from build123d import *

# Parameters (mm, degrees)
SKETCH_1_W          = 95.5
SKETCH_1_H          = 95.5
EXTRUDE_1_DEPTH     = 12
CUT_EXTRUDE_1_DEPTH = 69.58662406
FILLET_2_R          = 15
SKETCH_3_R          = 75
EXTRUDE_2_DEPTH     = 2
CHAMFER_1_SIZE      = 12
FILLET_1_R          = 1
SKETCH_6_W          = 42
SKETCH_6_H          = 42
CUT_EXTRUDE_3_DEPTH = 107.98598046
SKETCH_7_R          = 1.6
CUT_EXTRUDE_4_DEPTH = 107.98598046
CUT_EXTRUDE_5_DEPTH = 107.98598046
CUT_EXTRUDE_6_DEPTH = 0.5
SKETCH_10_W         = 12
SKETCH_10_H         = 12
CUT_EXTRUDE_7_DEPTH = 107.98598046
SKETCH_11_W         = 42
SKETCH_11_H         = 42
EXTRUDE_3_DEPTH     = 14
FILLET_3_R          = 2
SKETCH_12_W         = 41.3
SKETCH_12_H         = 41.3
CUT_EXTRUDE_8_DEPTH = 107.98598046
FILLET_4_R          = 5
SKETCH_13_R         = 3.25
CUT_EXTRUDE_9_DEPTH = 3


with BuildPart() as part:
    # ｽｹｯﾁ1 → ﾎﾞｽ - 押し出し1 (new body)
    with BuildSketch(Plane.XY):
        Rectangle(SKETCH_1_W, SKETCH_1_H)
    extrude(amount=EXTRUDE_1_DEPTH)

    # ｽｹｯﾁ2 → ｶｯﾄ - 押し出し1 (cut, through all)
    with BuildSketch(Plane.XY.offset(12)):
        Polygon((-16, 47.75), (-20, 20), (-47.75, 16), (-47.75, 47.75), align=None)
        Polygon((-16, -47.75), (-20, -20), (-47.75, -16), (-47.75, -47.75), align=None)
    cut_extrude_1 = extrude(amount=-CUT_EXTRUDE_1_DEPTH, mode=Mode.SUBTRACT)

    # ﾐﾗｰ1: ｶｯﾄ - 押し出し1 across plane
    add(cut_extrude_1.mirror(Plane(origin=(0, 0, 0), x_dir=(0, 0, 1), z_dir=(1, 0, 0))), mode=Mode.SUBTRACT)

    # ﾌｨﾚｯﾄ2
    fillet_2_edges = [part.edges().sort_by_distance(p)[0] for p in [
        (-20, 20, 6),
        (-20, -20, 6),
        (20, 20, 6),
        (20, -20, 6),
    ]]
    fillet(fillet_2_edges, radius=FILLET_2_R)

    # ｽｹｯﾁ3 → ﾎﾞｽ - 押し出し2 (add)
    with BuildSketch(Plane(origin=(0, 0, 0), x_dir=(-1, 0, 0), z_dir=(0, 0, -1))):
        Circle(SKETCH_3_R)
    extrude(amount=EXTRUDE_2_DEPTH)

    # 面取り1
    chamfer_1_edges = [part.edges().sort_by_distance(p)[0] for p in [
        (0, 47.75, 0),
        (47.75, 0, 0),
        (0, -47.75, 0),
        (-47.75, 0, 0),
    ]]
    chamfer(chamfer_1_edges, length=CHAMFER_1_SIZE - 0.0001)  # a hair under: the kernel refuses the full size

    # ﾌｨﾚｯﾄ1
    fillet_1_edges = [part.edges().sort_by_distance(p)[0] for p in [
        (75, 0, 0),
        (75, 0, -2),
    ]]
    fillet(fillet_1_edges, radius=FILLET_1_R - 0.0001)  # a hair under: the kernel refuses the full size

    # ｽｹｯﾁ6 → ｶｯﾄ - 押し出し3 (cut, through all)
    with BuildSketch(Plane.XY.offset(12)):
        Rectangle(SKETCH_6_W, SKETCH_6_H)
    extrude(amount=-CUT_EXTRUDE_3_DEPTH, mode=Mode.SUBTRACT)

    # ｽｹｯﾁ7 → ｶｯﾄ - 押し出し4 (cut, through all)
    with BuildSketch(Plane.XY.offset(12)):
        with Locations((0.15, 39.15)):
            Circle(SKETCH_7_R)
        with Locations((-39.15, 0.15)):
            Circle(SKETCH_7_R)
        with Locations((39.15, -0.15)):
            Circle(SKETCH_7_R)
        with Locations((-0.15, -39.15)):
            Circle(SKETCH_7_R)
    extrude(amount=-CUT_EXTRUDE_4_DEPTH, mode=Mode.SUBTRACT)

    # ｽｹｯﾁ8 → ｶｯﾄ - 押し出し5 (cut, through all)
    with BuildSketch(Plane(origin=(0, 0, -2), x_dir=(-1, 0, 0), z_dir=(0, 0, -1))):
        Polygon((-45.748737342, 53.526911935), (-46.809397513, 52.466251763), (-45.04163056, 50.69848481), (-43.980970389, 51.759144982), align=None)
        Polygon((-53.526911935, 45.748737342), (-51.759144982, 43.980970389), (-50.69848481, 45.04163056), (-52.466251763, 46.809397513), align=None)
        Polygon((43.980970389, 51.759144982), (45.04163056, 50.69848481), (46.809397513, 52.466251763), (45.748737342, 53.526911935), align=None)
        Polygon((51.759144982, 43.980970389), (53.526911935, 45.748737342), (52.466251763, 46.809397513), (50.69848481, 45.04163056), align=None)
    cut_extrude_5 = extrude(amount=-CUT_EXTRUDE_5_DEPTH, mode=Mode.SUBTRACT)

    # ｽｹｯﾁ9 → ｶｯﾄ - 押し出し6 (cut)
    with BuildSketch(Plane.XY):
        Polygon((-53.526911935, 45.748737342), (-45.748737342, 53.526911935), (-43.980970389, 51.759144982), (-51.759144982, 43.980970389), align=None)
        Polygon((43.980970389, 51.759144982), (51.759144982, 43.980970389), (53.526911935, 45.748737342), (45.748737342, 53.526911935), align=None)
    cut_extrude_6 = extrude(amount=-CUT_EXTRUDE_6_DEPTH, mode=Mode.SUBTRACT)

    # ﾐﾗｰ2: ｶｯﾄ - 押し出し5, ｶｯﾄ - 押し出し6 across plane
    add(cut_extrude_5.mirror(Plane.ZX), mode=Mode.SUBTRACT)
    add(cut_extrude_6.mirror(Plane.ZX), mode=Mode.SUBTRACT)

    # ｽｹｯﾁ10 → ｶｯﾄ - 押し出し7 (cut, through all)
    with BuildSketch(Plane.XY.offset(12)):
        with Locations((-29.75, 9.25)):
            Rectangle(SKETCH_10_W, SKETCH_10_H)
        with Locations((-9.25, -29.75)):
            Rectangle(SKETCH_10_W, SKETCH_10_H)
        with Locations((29.75, -9.25)):
            Rectangle(SKETCH_10_W, SKETCH_10_H)
        with Locations((9.25, 29.75)):
            Rectangle(SKETCH_10_W, SKETCH_10_H)
    extrude(amount=-CUT_EXTRUDE_7_DEPTH, mode=Mode.SUBTRACT)

    # ｽｹｯﾁ11 → ﾎﾞｽ - 押し出し3 (add, through all)
    with BuildSketch(Plane(origin=(0, 0, -2), x_dir=(-1, 0, 0), z_dir=(0, 0, -1))):
        Rectangle(SKETCH_11_W, SKETCH_11_H)
    extrude(amount=-EXTRUDE_3_DEPTH)

    # ﾌｨﾚｯﾄ3
    fillet_3_edges = [part.edges().sort_by_distance(p)[0] for p in [
        (-35.75, 3.25, 5),
        (-35.75, 15.25, 5),
        (-23.75, 15.25, 5),
        (-23.75, 3.25, 5),
        (-15.25, -35.75, 5),
        (-15.25, -23.75, 5),
        (-3.25, -23.75, 5),
        (-3.25, -35.75, 5),
        (35.75, -3.25, 5),
        (35.75, -15.25, 5),
        (23.75, -15.25, 5),
        (23.75, -3.25, 5),
        (15.25, 35.75, 5),
        (15.25, 23.75, 5),
        (3.25, 23.75, 5),
        (3.25, 35.75, 5),
    ]]
    fillet(fillet_3_edges, radius=FILLET_3_R)

    # ｽｹｯﾁ12 → ｶｯﾄ - 押し出し8 (cut, through all)
    with BuildSketch(Plane.XY.offset(12)):
        Rectangle(SKETCH_12_W, SKETCH_12_H)
    extrude(amount=-CUT_EXTRUDE_8_DEPTH, mode=Mode.SUBTRACT)

    # ﾌｨﾚｯﾄ4
    fillet_4_edges = [part.edges().sort_by_distance(p)[0] for p in [
        (-20.65, -20.65, 5),
        (-20.65, 20.65, 5),
        (20.65, 20.65, 5),
        (20.65, -20.65, 5),
    ]]
    fillet(fillet_4_edges, radius=FILLET_4_R)

    # ｽｹｯﾁ13 → ｶｯﾄ - 押し出し9 (cut)
    with BuildSketch(Plane(origin=(0, 0, -2), x_dir=(-1, 0, 0), z_dir=(0, 0, -1))):
        with Locations((-0.15, 39.15)):
            Circle(SKETCH_13_R)
        with Locations((39.15, 0.15)):
            Circle(SKETCH_13_R)
        with Locations((-39.15, -0.15)):
            Circle(SKETCH_13_R)
        with Locations((0.15, -39.15)):
            Circle(SKETCH_13_R)
    extrude(amount=-CUT_EXTRUDE_9_DEPTH, mode=Mode.SUBTRACT)


solid = part.part
The listing builds one solid part. Answer for the finished solid, in the listing's coordinates (mm). A direction names the side the tool comes from. Coordinates: 2 decimals unless noted, no trailing zeros. Answer in a Markdown table with one row per item. Add a question column.
1. Determine the mould class of faces 4 (the flat face through (-22, 1, 12)), 5 (the flat face through (-9, -35.75, 5)), 6 (the flat face through (53.67, -0.22, 6.08)) for opening direction X: +X half, -X half, draft (parallel to the pull), parting line (faces both ways), or undercut.
2. The part is cut by section A-A, the plane y = -11. Count the separate pieces of the cut face and the enclosed holes in it, then the cut area to 3 significant figures.
3. For faces 1 (the cylindrical face through (-3.25, -38.17, -0.52)), 2 (the cylindrical face through (-22.735, -22.544, 5.916)), 3 (the flat face through (9, 23.75, 5)), determine the directions among +Z, -Z, +X, -X, +Y, -Y from which every point of the face is accessible in a straight line to the end or side of a thin tool.
4. Flat-ended cylindrical pins translate along their axes: P1, Ø6.5, axis at x = 28, z = 5.5, coming from the -Y side; P2, Ø8, axis at y = 53.5, z = 7.5, coming from the -X side; P3, Ø7, axis at x = -38, y = 0.5, coming from the -Z side; P4, Ø6.5, axis at y = -10.5, z = 7.5, coming from the +X side. Find the tip coordinate at first contact, or state that the pin passes through.
5. Consider line 1 (Y direction, x = 0.15, z = 5); line 2 (Y direction, x = 53, z = -0.25); line 3 (Y direction, x = 0.15, z = 6.5). Determine where each line is inside the solid, lowest interval first. Write a range as [from, to].
Answer below:
| question | item | result |
|---|---|---|
| 1 | face 4 | draft |
| 1 | face 5 | undercut |
| 1 | face 6 | +X half |
| 2 | separate pieces | 3 |
| 2 | enclosed holes | 0 |
| 2 | area | 840 mm2 |
| 3 | face 1 | -Z |
| 3 | face 2 | +Z, -X, -Y |
| 3 | face 3 | +Z, -Z |
| 4 | P1 | y = -20.88 |
| 4 | P2 | x = -15.75 |
| 4 | P3 | z = -2 |
| 4 | P4 | x = 55.5 |
| 5 | line 1 | [-54.75, -40.72], [-37.58, -20.65], [20.65, 37.55], [40.75, 54.75] |
| 5 | line 2 | [-52.59, -46.28], [-45.22, 45.22], [46.28, 52.59] |
| 5 | line 3 | [-53.25, -40.72], [-37.58, -20.65], [20.65, 37.55], [40.75, 53.25] |
